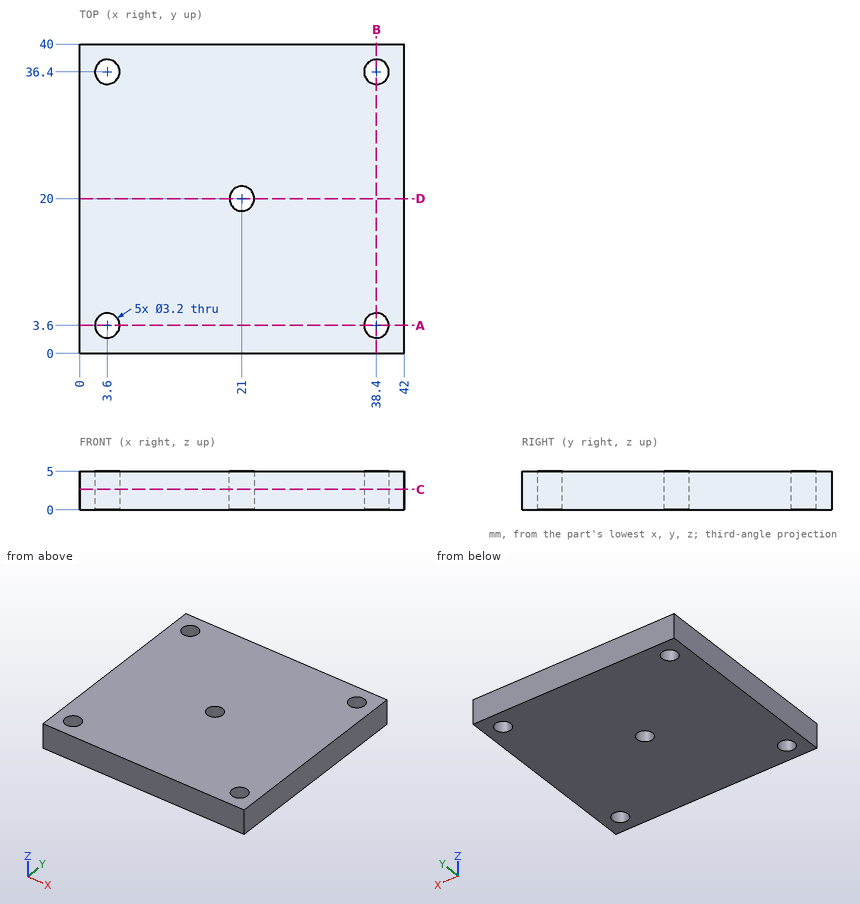
Drawing for the job (mm, zero at the part's lowest x, y, z). Give positions to 0.01 mm unless a question says otherwise; leave off trailing zeros. Order: outer loops, then holes, each group sorted by start corner. A loop starts at its lowest first (then second) coordinate and runs counter-clockwise, first axis right, second up. Notation, with made-up numbers: M 65.5,66 L 123.5,66 A20 ccw 123.5,84 Z; hole C 76.25,3 d10. An arc over 180 degrees is marked long. Use a Markdown table: item, result. Add a question column.
(1) Drop a flat-ended pin along its axis: P1, Ø1.9, axis at x = 38.4, y = 36.4, coming from the +Z side. Give the stop position or say it passes through.
(2) Saw through at A-A, the plane y = 3.6. Give the cut face in (x, z), and give its area (3 significant figures).
(3) Saw through at C-C, the plane z = 2.65. Give the cut face in (x, y).
(4) Saw through at D-D, the plane y = 20. Give the cut face in (x, z).
(5) Saw through at B-B, the plane x = 38.4. Give the cut face in (y, z), and give its area (3 significant figures).
(6) Probe line 1 along Y through (x, z) = (38.4, 1.55); line 2 along X through (y, z) = (2.5, 1.15); line 3 along X through (y, z) = (4, 3.7). List the from-to ranges inside material, lowest first. Write a range as [from, to].
Answer key:
| question | item | result |
|---|---|---|
| 1 | P1 | through |
| 2 | outline | M 0,0 L 2,0 L 2,5 L 0,5 Z; M 5.2,0 L 36.8,0 L 36.8,5 L 5.2,5 Z; M 40,0 L 42,0 L 42,5 L 40,5 Z |
| 2 | area | 178 mm^2 |
| 3 | outline | M 0,0 L 42,0 L 42,40 L 0,40 Z; hole C 3.6,3.6 d3.2; hole C 3.6,36.4 d3.2; hole C 21,20 d3.2; hole C 38.4,3.6 d3.2; hole C 38.4,36.4 d3.2 |
| 4 | outline | M 0,0 L 19.4,0 L 19.4,5 L 0,5 Z; M 22.6,0 L 42,0 L 42,5 L 22.6,5 Z |
| 5 | outline | M 0,0 L 2,0 L 2,5 L 0,5 Z; M 5.2,0 L 34.8,0 L 34.8,5 L 5.2,5 Z; M 38,0 L 40,0 L 40,5 L 38,5 Z |
| 5 | area | 168 mm^2 |
| 6 | line 1 | [0, 2], [5.2, 34.8], [38, 40] |
| 6 | line 2 | [0, 2.44], [4.76, 37.24], [39.56, 42] |
| 6 | line 3 | [0, 2.05], [5.15, 36.85], [39.95, 42] |
